Design review of the part built by this model. Coordinates are the model's own, in mm. Face numbers are marked on the shaded views. A direction names the side the tool comes from. Give positions to 0.01 mm unless a question says otherwise; leave off trailing zeros. Order: outer loops, then holes, each group sorted by start corner. A loop starts at its lowest first (then second) coordinate and runs counter-clockwise, first axis right, second up. Notation, with made-up numbers: (-27.75, 75) -> (22.25, 75) arc R25 ccw to (22.25, 94) -> close; hole circle Ø11 at (27, 84.25). An arc over 180 degrees is marked (long way). Use a Markdown table: item, result. Add a question column.
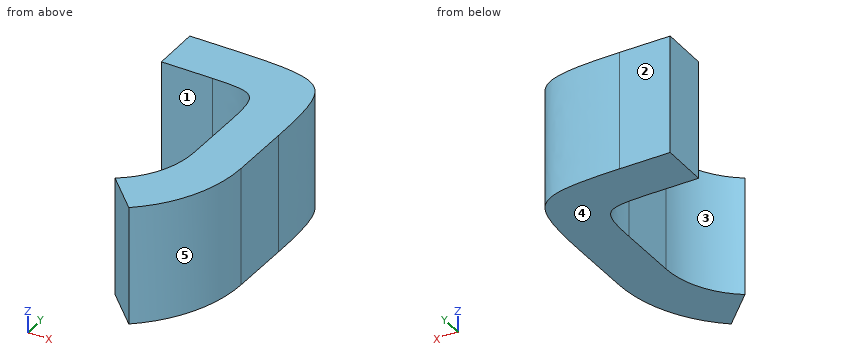
```python
from build123d import *

# Parameters (mm, degrees)
F3_DEPTH    = 5
F4_T1_DEPTH = 5
F5_T1_DEPTH = 25.3094755674


# Not quite as in the source:
# - a fillet or chamfer that OpenCascade refuses, or shapes differently, is made with other operations: its cross-section is extruded or revolved along the edge and cut away or added
# - a feature of the source that left no trace in its solid (it failed there, or was rolled back) is left out


with BuildPart() as f3:
    # F2 (on Top) → F3 (new body)
    with BuildSketch(Plane.XY):
        with BuildLine():
            Line((5.5017601699, 0), (5.5017601699, -2))
            Line((5.5017601699, -2), (9.6698484997, -2))
            Line((9.6698484997, -2), (9.5995756294, -6.5762830432))
            ThreePointArc((9.5995756294, -6.5762830432), (9.167895168, -8.2311078505), (8.0212889249, -9.5))
            Line((8.0212889249, -9.5), (9.4518866721, -10.9305977473))
            ThreePointArc((9.4518866721, -10.9305977473), (11.0154330705, -9.0120786534), (11.5993398679, -6.6069911903))
            Line((11.5993398679, -6.6069911903), (11.7007960564, 0))
            Line((11.7007960564, 0), (5.5017601699, 0))
        make_face()
    extrude(amount=F3_DEPTH)

    # F4: fillet of radius 2 on 1 edges, made by hand

    # F4_s2 → F4_t1 (join)
    with BuildSketch(Plane.XY):
        with BuildLine():
            add(Edge.make_bspline(
                [(7.638900943, -2), (9.6698484997, -2), (9.6386651815, -4.0307081471)],
                knots=[0, 0, 0, 1, 1, 1], degree=2, weights=[1, 2.3333333333, 1]))
            Line((9.6386651815, -4.0307081471), (9.6698484997, -2))
            Line((9.6698484997, -2), (7.638900943, -2))
        make_face()
    extrude(amount=F4_T1_DEPTH)

    # F5: fillet of radius 4 on 1 edges, made by hand

    # F5_s2 → F5_t1 (cut)
    with BuildSketch(Plane.XY.offset(-10.1547377837)):
        with BuildLine():
            add(Edge.make_bspline(
                [(11.63842942, -4.0614162943), (11.7007960564, 0), (7.638900943, 0)],
                knots=[0, 0, 0, 1, 1, 1], degree=2, weights=[1, 2.3333333333, 1]))
            Line((7.638900943, 0), (11.7007960564, 0))
            Line((11.7007960564, 0), (11.63842942, -4.0614162943))
        make_face()
    extrude(amount=F5_T1_DEPTH, mode=Mode.SUBTRACT)


solid = f3.part
```
1) Insertion check: pin 1 (1.1 mm diameter, centred on x = 6, z = 2.5, fed in from -Y); pin 2 (3 mm diameter, centred on x = 9, y = -7.5, fed in from +Z). Each pin has a flat end and moves straight along its axis. Give the tip position at first contact, or say it passes through.
2) Add section A-A (x = 7.25). Give the boundary of the cut face in (y, z), then the cut area to 3 significant figures.
3) The part is to be moulded in two halves that separate along Y. For the marked faces 3, 4 and 5, say which applies: +Y half, -Y half, draft (parallel to the pull), parting line (faces both ways), or undercut.
4) Add section B-B (y = -10). Give the boundary of the cut face in (x, z), then the cut area to 3 significant figures.
5) Machinability: for the marked faces 1 and 2, which of the approach directions +Z, -Z, +X, -X, +Y, -Y give a long, thin tool a straight path to every point of the face, cutting with its end or side? Answer none if there is none.
6) For L1, parallel to X at y = -6.5, z = 2.65; L2, parallel to Y at x = 6.5, z = 2.95; L3, parallel to Y at x = 8.25, z = 2.3, list the stretches that pass through material, from the lowest coordinate up. Write a range as [from, to].
Worked answers:
| question | item | result |
|---|---|---|
| 1 | pin 1 | y = -2 |
| 1 | pin 2 | z = 5 |
| 2 | outline | (-2, 0) -> (0, 0) -> (0, 5) -> (-2, 5) -> close |
| 2 | area | 10.0 mm^2 |
| 3 | face 3 | undercut |
| 3 | face 4 | draft |
| 3 | face 5 | -Y half |
| 4 | outline | (8.52, 0) -> (10.39, 0) -> (10.39, 5) -> (8.52, 5) -> close |
| 4 | area | 9.33 mm^2 |
| 5 | face 1 | +Z, -Z, -X, -Y |
| 5 | face 2 | +Z, -Z, +X, -X, +Y |
| 6 | L1 | [9.6, 11.6] |
| 6 | L2 | [-2, 0] |
| 6 | L3 | [-9.73, -9.33], [-2.01, 0] |
